Autodesk Inventor part; units mm, degrees
ref_plane "YZ Plane" through (0, 0, 0) normal (1, 0, 0) x (0, 1, 0)
ref_plane "XZ Plane" through (0, 0, 0) normal (0, 1, 0) x (-1, 0, 0)
ref_plane "XY Plane" through (0, 0, 0) normal (0, 0, 1) x (1, 0, 0)
sketch "Sketch1" plane through (0, 0, 0) normal (1, 0, 0) x (0, 1, 0)
  line L0 (0, 0) -> (-15.875, 0)
  line L1 (-15.875, 0) -> (-15.875, -20.32)
  line L2 (-15.875, -20.32) -> (-5.461, -20.32)
  line L3 (-5.461, -20.32) -> (-5.461, -8.636)
  line L4 (-5.461, -8.636) -> (0, -8.636)
  line L5 (0, -8.636) -> (0, 0)
  dimension "d0" = 15.875
  dimension "d1" = 10.414
  dimension "d2" = 20.32
  dimension "d3" = 8.636
revolve "Revolution1" add sketch "Sketch1" angle 360 about axis through (0, 0, 0) along (0, -1, 0)
sketch "Sketch3" plane through (0, 0, 0) normal (0, 1, 0) x (1, 0, 0)
  line L0 (0, -31.0012) -> (0, 35.3144)
  line L1 (-32.7265, 0) -> (26.1488, 0)
  point P0 (0, 0)
  point P1 (-14.2875, 0)
  point P2 (0, 0)
  point P3 (0, 14.2875)
  point P4 (14.2875, 0)
  point P5 (0, -14.2875)
  dimension "d23" = 28.575
  dimension "d24" = 28.575
hole "Hole3" at (0, 0, 0) direction (0, -1, 0) diameter 10 end through all
hole "Hole4" at (0, 0, -14.2875) at (-14.2875, 0, 0) at (0, 0, 14.2875) at (14.2875, 0, 0) direction (0, -1, 0) diameter 6.7564 end through all
properties part number "Flange_Nut_7549K16"
Check sheet for the modelled part. Datum: model origin and axes. Units: mm. A direction names the side the tool comes from. Coordinates: 2 decimals unless noted, no trailing zeros. Order: outer loops, then holes, each group sorted by start corner. A loop starts at its lowest first (then second) coordinate and runs counter-clockwise, first axis right, second up. Notation, with made-up numbers: (6.25, -24) -> (36.25, -24) arc R14 ccw to (36.25, -6) -> close; hole circle Ø5 at (22.5, 18.25). An arc over 180 degrees is marked (long way). Write item = value, one per line. Start each with the question number.
1) Material ranges on L1, parallel to X at y = -11.25, z = 0; L2, parallel to Z at x = 0.5, y = -11; L3, parallel to Y at x = -13, z = -8.5 (3 decimals), recorded low to high.
2) Cross-section at D-D (x = -4.5). Enter the section's corners in (y, z) (3 decimals), then the cut area to 3 significant figures.
3) Cross-section at B-B (z = 0). Enter the section's corners in (x, y) (3 decimals), then the cut area to 3 significant figures.
4) Cross-section at A-A (x = 0). Enter the section's corners in (y, z) (3 decimals), then the cut area to 3 significant figures.
5) Mould release check, pull along X, two halves, no side actions. Record for faces 3 (the cylindrical face through (-20.147, -10.595, 2.645)), 4 (the cylindrical face through (4.88, -8.05, -1.08)), 5 (the flat face through (-4, -15.875, -4)), 6 (the cylindrical face through (-1.01, -10.74, 17.51)): +X half, -X half, draft (parallel to the pull), parting line (faces both ways), or undercut.
6) Cross-section at C-C (z = 16). Enter the section's corners in (x, y) (3 decimals).
7) Access from +Z, -Z, +X, -X, +Y, -Y to the whole of each face (thin tool, end or side, straight path). Record for faces 1 (the flat face through (-4, 0, -4)), 2 (the flat face through (-9, -5.461, 0)).
8) Go/stop test with flat-tipped pins: P1, Ø6, axis at x = 1, y = -2, coming from the +Z side; P2, Ø6, axis at x = 15, y = -9.5, coming from the +Z side; P3, Ø16, axis at x = 0, z = 0, coming from the -Y side (3 decimals); P4, Ø1, axis at x = -11, y = -8.5, coming from the -Z side. Record where each tip stops, or that it passes through.
Ans:
q1.L1 = -20.32 to -17.67, -10.91 to -5, 5 to 10.91, 17.67 to 20.32
q1.L2 = -20.31 to -17.63, -10.95 to -4.97, 4.97 to 10.95, 17.63 to 20.31
q1.L3 = -15.875 to -5.461
q2.outline = (-15.875, -19.815) -> (-5.461, -19.815) -> (-5.461, -7.371) -> (0, -7.371) -> (0, -2.179) -> (-15.875, -2.179) -> close; (-15.875, 2.179) -> (0, 2.179) -> (0, 7.371) -> (-5.461, 7.371) -> (-5.461, 19.815) -> (-15.875, 19.815) -> close
q2.area = 424 mm²
q3.outline = (-20.32, -15.875) -> (-17.666, -15.875) -> (-17.666, -5.461) -> (-20.32, -5.461) -> close; (-10.909, -15.875) -> (-5, -15.875) -> (-5, 0) -> (-8.636, 0) -> (-8.636, -5.461) -> (-10.909, -5.461) -> close; (5, -15.875) -> (10.909, -15.875) -> (10.909, -5.461) -> (8.636, -5.461) -> (8.636, 0) -> (5, 0) -> close; (17.666, -15.875) -> (20.32, -15.875) -> (20.32, -5.461) -> (17.666, -5.461) -> close
q3.area = 218 mm²
q4.outline = (-15.875, -20.32) -> (-5.461, -20.32) -> (-5.461, -17.666) -> (-15.875, -17.666) -> close; (-15.875, -10.909) -> (-5.461, -10.909) -> (-5.461, -8.636) -> (0, -8.636) -> (0, -5) -> (-15.875, -5) -> close; (-15.875, 5) -> (0, 5) -> (0, 8.636) -> (-5.461, 8.636) -> (-5.461, 10.909) -> (-15.875, 10.909) -> close; (-15.875, 17.666) -> (-5.461, 17.666) -> (-5.461, 20.32) -> (-15.875, 20.32) -> close
q4.area = 218 mm²
q5.face_3 = parting line
q5.face_4 = undercut
q5.face_5 = draft
q5.face_6 = undercut
q6.outline = (-12.526, -15.875) -> (-2.912, -15.875) -> (-2.912, -5.461) -> (-12.526, -5.461) -> close; (2.912, -15.875) -> (12.526, -15.875) -> (12.526, -5.461) -> (2.912, -5.461) -> close
q7.face_1 = +Z, -Z, +X, -X, +Y
q7.face_2 = +Y
q8.P1 = 8.64
q8.P2 = 16.4
q8.P3 = -15.875
q8.P4 = -17.4
